The listing builds one solid part. Answer for the finished solid, in the listing's coordinates (mm). Face numbers are marked on the shaded views. Give positions to 0.01 mm unless a question says otherwise; leave off trailing zeros. Write each loop counter-clockwise with the first axis right and the second up, starting at its lowest first coordinate (ties: lowest second). Pieces come first, ordered by that corner, then holes. Notation, with made-up numbers: (-37, 60) - (7, 60) arc R19 cw to (7, 65) - close; hole circle Ø8 at (10, 49.5). An arc over 180 degrees is marked (long way). Return JSON: item names as keys, results as strings.
from build123d import *

# Parameters (mm, degrees)
F1_W     = 25.4
F1_H     = 25.2323417494
F2_DEPTH = 25.4
F3_R     = 6.35
F4_DEPTH = 16.9333333333


# Not quite as in the source:
# - the program builds the solid bodies; features that only make, move or delete a surface that nothing else refers to are left out


with BuildPart() as f2:
    # F1 (on Front) → F2 (new body)
    with BuildSketch(Plane.XZ):
        Polygon((12.7, 39.5754580502), (0, 25.2323417494), (25.4, 25.2323417494), align=None)
        with Locations((12.7, 12.6161708747)):
            Rectangle(F1_W, F1_H)
    extrude(amount=-F2_DEPTH)

    # F3 (on face) → F4 (cut)
    with BuildSketch(Plane.XZ):
        with Locations((12.7, 14.1754580502)):
            Circle(F3_R)
    extrude(amount=-F4_DEPTH, mode=Mode.SUBTRACT)


solid = f2.part
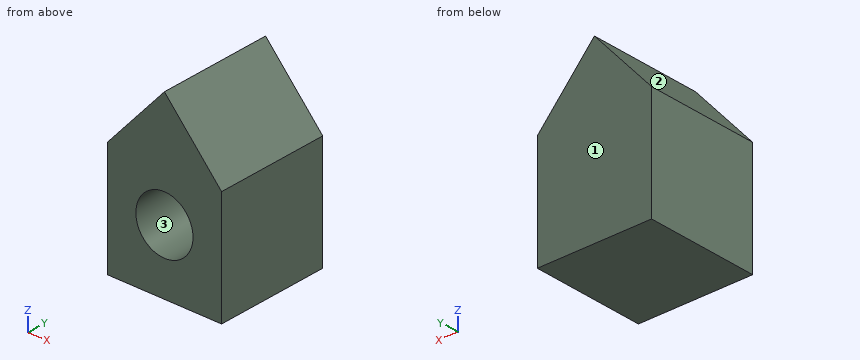
Item 1: A cutting plane is placed at D-D on z = 13. Determine the outline of the cut face in (x, y).
Answer below:
{"outline": "(0, 0) - (6.46, 0) - (6.46, 16.93) - (18.94, 16.93) - (18.94, 0) - (25.4, 0) - (25.4, 25.4) - (0, 25.4) - close"}
Item 2: A cutting plane is placed at A-A on x = 12.25. Determine the outline of the cut face in (y, z).
Answer below:
{"outline": "(0, 0) - (25.4, 0) - (25.4, 39.07) - (0, 39.07) - (0, 20.51) - (16.93, 20.51) - (16.93, 7.84) - (0, 7.84) - close"}
Item 3: Flat-ended cylindrical pins translate along their axes: P1, Ø6.5, axis at x = 13, z = 15, coming from the -Y side; P2, Ø5, axis at x = 9.5, y = 13.5, coming from the +Z side. Find the tip coordinate at first contact, or state that the pin passes through.
Answer below:
{"P1": "stops at y = 16.93", "P2": "stops at z = 38.78"}
Item 4: Consider L1, parallel to Y at x = 9.75, z = 9; L2, parallel to X at y = 10, z = 17.5; L3, parallel to X at y = 9.25, z = 34. Determine where each line is inside the solid, lowest interval first.
Answer below:
{"L1": "y = 16.93 to 25.4", "L2": "x = 0 to 7.29, 18.11 to 25.4", "L3": "x = 7.76 to 17.64"}
Item 5: A cutting plane is placed at C-C on y = 7.25. Determine the outline of the cut face in (x, z).
Answer below:
{"outline": "(0, 0) - (25.4, 0) - (25.4, 25.23) - (12.7, 39.58) - (0, 25.23) - close; hole circle Ø12.7 at (12.7, 14.18)"}
Item 6: A cutting plane is placed at B-B on y = 21.75. Determine the outline of the cut face in (x, z), then the cut area to 3 significant figures.
Answer below:
{"outline": "(0, 0) - (25.4, 0) - (25.4, 25.23) - (12.7, 39.58) - (0, 25.23) - close", "area": "823 mm²"}
Item 7: The mould has two halves that part along Z. Classify the marked faces 1, 2 and 3: +Z half, -Z half, draft (parallel to the pull), parting line (faces both ways), or undercut.
Answer below:
{"face 1": "draft", "face 2": "+Z half", "face 3": "undercut"}
